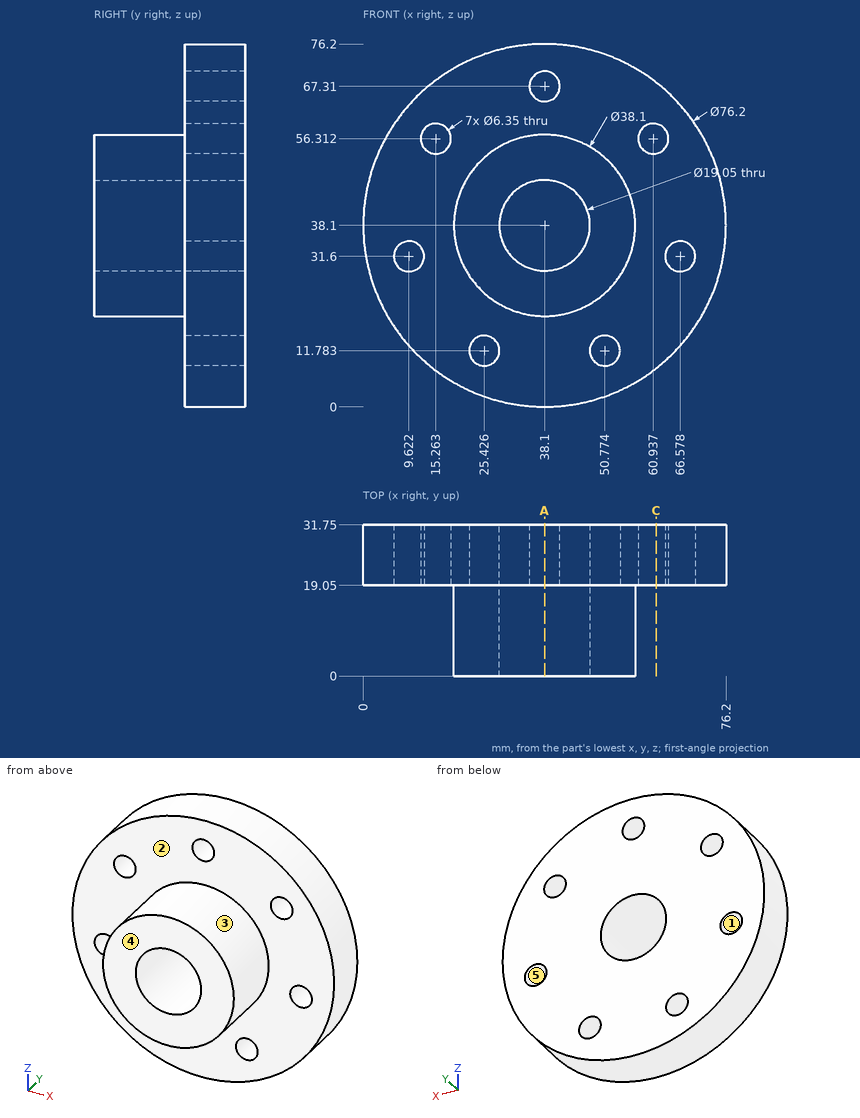
Could you check a few things on this drawing? It's one solid part, dimensions in mm from its lowest x, y, z. A direction names the side the tool comes from. Coordinates: 2 decimals unless noted, no trailing zeros. Loops run counter-clockwise (first coordinate to the right, second up) from the corner with the lowest first, then second, coordinate; pieces in that order, holes last. Notation, with made-up numbers: (-18, 20) - (27, 20) arc R20 cw to (27, 39) - close; hole circle Ø5 at (15.25, 80.5). An arc over 180 degrees is marked (long way). Return JSON: item names as keys, results as strings. Group by question number.
Item 1: Will these pins go through, and if not, where does the flat tip stop? P1, Ø5.5, axis at x = 25.43, z = 11.78, coming from the +Y side; P2, Ø2, axis at y = 27.5, z = 32, coming from the -X side; P3, Ø8.5, axis at x = 66.58, z = 31.6, coming from the +Y side; P4, Ø5, axis at y = 19, z = 61.5, coming from the +X side (1 decimal).
Item 2: We'd pull the mould along X, two halves only. Please class the marked faces 3, 4 and 5: +X half, -X half, draft (parallel to the pull), parting line (faces both ways), or undercut.
Item 3: On a 3-axis mill with a long thin cutter (end or side, diameter ignored), from which of +Z, -Z, +X, -X, +Y, -Y can I reach the whole of each face in a straight line? I mean the marked faces 1 and 2. Say none if no direction works.
Item 4: If we section it at C-C on x = 61.5: Write out the boundary of the cut face in (y, z), and give its area (3 significant figures).
Item 5: I need wall thicknesses on line 1 (X direction, y = 22.5, z = 12.5) (1 decimal); line 2 (Y direction, x = 26, z = 15); line 3 (X direction, y = 7.5, z = 43.5) (1 decimal). Which ranges of each line are inside material? Lowest first, please. Write a range as from..to.
Item 6: If we section it at A-A on x = 38.1: State how many separate pieces and enclosed holes the cut face has, and give its area (3 significant figures).
Calculated:
{
 "1": {"P1": "passes through", "P2": "stops at x = 0.34", "P3": "stops at y = 31.75", "P4": "stops at x = 70"},
 "2": {"face 3": "parting line", "face 4": "draft", "face 5": "undercut"},
 "3": {"face 1": "+Y, -Y", "face 2": "-Y"},
 "4": {"outline": "(19.05, 8.03) - (31.75, 8.03) - (31.75, 53.19) - (19.05, 53.19) - close; (19.05, 59.44) - (31.75, 59.44) - (31.75, 68.17) - (19.05, 68.17) - close", "area": "684 mm^2"},
 "5": {"line 1": "x = 9.9..22.3, 28.5..47.7, 53.9..66.3", "line 2": "y = 19.05..31.75", "line 3": "x = 19.8..30.3, 45.9..56.4"},
 "6": {"separate pieces": "3", "enclosed holes": "0", "area": "1,010 mm^2"}
}
